from build123d import *

# Parameters (mm, degrees)
EXTRUSION1_DEPTH        = 25
ENL_V_MAT_EXTRU_1_DEPTH = 4
ENL_V_MAT_EXTRU_2_DEPTH = 4.0000001
CONG_1_R                = 0.5


with BuildPart() as part:
    # Esquisse1 → Extrusion1 (new body, symmetric)
    with BuildSketch(Plane(origin=(0, 0, 0), x_dir=(1, 0, 0), z_dir=(0, 1, 0))):
        with BuildLine():
            Line((-1.5, 38.883399735), (-1.5, -38.883399735))
            ThreePointArc((-1.5, -38.883399735), (0, -38.75), (1.5, -38.883399735))
            Line((1.5, -38.883399735), (1.5, 38.883399735))
            ThreePointArc((1.5, 38.883399735), (0, 38.75), (-1.5, 38.883399735))
        make_face()
    extrude(amount=EXTRUSION1_DEPTH, both=True)

    # Esquisse2 → Enlèv. mat.-Extru.1 (cut, through all)
    with BuildSketch(Plane(origin=(1.5, 0, 0), x_dir=(0, 0, -1), z_dir=(1, 0, 0))):
        with BuildLine():
            Line((-33.883399735, 9), (-33.883399735, -9))
            ThreePointArc((-33.883399735, -9), (-35.347865829, -12.535533906), (-38.883399735, -14))
            Line((-38.883399735, -14), (-38.883399735, 14))
            ThreePointArc((-38.883399735, 14), (-35.347865829, 12.535533906), (-33.883399735, 9))
        make_face()
        with BuildLine():
            Line((38.883399735, 14), (38.883399735, -14))
            ThreePointArc((38.883399735, -14), (35.347865829, -12.535533906), (33.883399735, -9))
            Line((33.883399735, -9), (33.883399735, 9))
            ThreePointArc((33.883399735, 9), (35.347865829, 12.535533906), (38.883399735, 14))
        make_face()
        with BuildLine():
            Line((-38.883399735, 25), (38.883399735, 25))
            ThreePointArc((38.883399735, 25), (0, 17.5), (-38.883399735, 25))
        make_face()
        with BuildLine():
            Line((-38.883399735, -25), (38.883399735, -25))
            ThreePointArc((38.883399735, -25), (0, -17.5), (-38.883399735, -25))
        make_face()
    extrude(amount=-ENL_V_MAT_EXTRU_1_DEPTH, mode=Mode.SUBTRACT)

    # Esquisse3 → Enlèv. mat.-Extru.2 (cut, through all)
    with BuildSketch(Plane(origin=(1.5, 0, 0), x_dir=(0, 0, -1), z_dir=(1, 0, 0))):
        with BuildLine():
            Line((12.961481397, 1), (-12.961481397, 1))
            ThreePointArc((-12.961481397, 1), (-12.609240952, -3.163390997), (-10.95445115, -7))
            ThreePointArc((-10.95445115, -7), (0.529660497, -2.111220787), (12.961481397, -1))
            ThreePointArc((12.961481397, -1), (13, 0), (12.961481397, 1))
        make_face()
        with BuildLine():
            ThreePointArc((-7.350889359, 10.722146503), (2.043285167, 5.292013474), (12.649110641, 3))
            ThreePointArc((12.649110641, 3), (4.682485861, 12.127420425), (-7.350889359, 10.722146503))
        make_face()
        with BuildLine():
            ThreePointArc((12.649110641, -3), (2.457687621, -4.516686577), (-4.350889359, -12.250296396))
            ThreePointArc((-4.350889359, -12.250296396), (6.213462397, -11.418970402), (12.649110641, -3))
        make_face()
    extrude(amount=-ENL_V_MAT_EXTRU_2_DEPTH, mode=Mode.SUBTRACT)

    # Congé1
    cong_1_edges = [part.edges().sort_by_distance(p)[0] for p in [
        (-1.5, 17.5, 0),
        (1.5, 17.5, 0),
        (-1.5, -17.5, 0),
        (1.5, -17.5, 0),
        (-1.5, 12.535533906, 35.347865829),
        (-1.5, -12.535533906, 35.347865829),
        (-1.5, 0, 33.883399735),
        (1.5, 12.535533906, 35.347865829),
        (1.5, -12.535533906, 35.347865829),
        (1.5, 0, 33.883399735),
        (-1.5, -12.535533906, -35.347865829),
        (-1.5, 12.535533906, -35.347865829),
        (-1.5, 0, -33.883399735),
        (1.5, -12.535533906, -35.347865829),
        (1.5, 12.535533906, -35.347865829),
        (1.5, 0, -33.883399735),
    ]]
    fillet(cong_1_edges, radius=CONG_1_R)


solid = part.part
Could you check a few things on this model? Use its own coordinates, in mm. A direction names the side the tool comes from. Round coordinates to 2 decimals unless told otherwise and drop trailing zeros. Write each loop counter-clockwise with the first axis right and the second up, starting at its lowest first coordinate (ties: lowest second). Pieces come first, ordered by that corner, then holes. Notation, with made-up numbers: (55, 13) - (59, 13) arc R18 ccw to (59, 31) - close; hole circle Ø2 at (-34, 36.25). An arc over 180 degrees is marked (long way). Put each result on its own line as item: value. Start each with the question number.
(1) I want a section at A-A, the plane x = -0.1. Please give me the cut outline in (y, z), plus the area to 3 significant figures.
(2) For faces 1 (the cylindrical face through (0.01, -12.55, -35.36)), 2 (the cylindrical face through (0.02, 19.56, -38.75)), 3 (the cylindrical face through (0.01, 12.55, 35.36)), 4 (the flat face through (1.5, 6, 1)), 5 (the cylindrical face through (0, 0, -13)), which set-ups out of +Z, -Z, +X, -X, +Y, -Y let a thin tool reach every point of the face, with its end or its side?
(3) I want a section at B-B, the plane z = -3.5. Give the number of separate pieces and of enclosed holes in the cut face, plus the area to 3 significant figures.
(4) Thinking about a two-plate mould opening in Y: for faces 6 (the flat face through (0, 0, 33.883)), 7 (the cylindrical face through (0, -17.5, -0.6)), 8 (the cylindrical face through (-0.02, -19.41, 38.75)), 9 (the cylindrical face through (0, 17.5, -0.6)), which applies, released by +Y, released by -Y, zero draft, split by the parting line, or undercut?
(5) I need wall thicknesses on probe 1 along Z at (x, y) = (0.35, -6.5); probe 2 along Z at (x, y) = (0.6, -4.5); probe 3 along Y at (x, z) = (0.2, 3). Which ranges of each line are inside material? Lowest first, please.
(6) Will these pins go through, and if not, where does the flat tip stop? pin 1 (1 mm diameter, centred on x = 0.5, y = -8.5, fed in from -Z); pin 2 (1 mm diameter, centred on x = 0.5, y = -4, fed in from +Z).
Here are the results:
1. outline: (-24.95, -38.75) - (-14, -38.75) arc R5 cw to (-9, -33.88) - (9, -33.88) arc R5 cw to (14, -38.75) - (24.95, -38.75) arc R104.54 cw to (24.95, 38.75) - (14, 38.75) arc R5 cw to (9, 33.88) - (-9, 33.88) arc R5 cw to (-14, 38.75) - (-24.95, 38.75) arc R104.54 cw to start; hole (-12.25, 4.35) arc R13 ccw to (-3, -12.65) arc R15 ccw to start; hole (-7, 10.95) arc R40 cw to (-1, -12.96) arc R13 ccw to (1, -12.96) - (1, 12.96) arc R13 ccw to start; hole (3, -12.65) arc R13 ccw to (10.72, 7.35) arc R35 ccw to start
1. area: 2,530 mm^2
2. face 1: -Z, +X, -X
2. face 2: -Z, +Y, -Y
2. face 3: +Z, +X, -X
2. face 4: +Z, -Z, +X, +Y, -Y
2. face 5: +X, -X
3. separate pieces: 4
3. enclosed holes: 0
3. area: 48.9 mm^2
4. face 6: undercut
4. face 7: released by -Y
4. face 8: zero draft
4. face 9: released by +Y
5. probe 1: z = -33.88 to -11.26, 0.36 to 10.13, 11.26 to 33.88
5. probe 2: z = -33.88 to -12.2, -2.49 to 6.3, 12.2 to 33.88
5. probe 3: y = -17.54 to -12.65, -9.6 to -3.17, 1 to 7.72, 12.65 to 17.54
6. pin 1: stops at z = -33.88
6. pin 2: stops at z = 33.88
